Part model, mm, in its own coordinate system. A direction names the side the tool comes from. Round coordinates to 2 decimals unless told otherwise and drop trailing zeros. Loops run counter-clockwise (first coordinate to the right, second up) from the corner with the lowest first, then second, coordinate; pieces in that order, holes last.
(1) Cut at D-D on x = -4. List the corners of the cut face in (y, z).
(2) Mould opens along Z. For faces 1 (the face through (0, 15, -15)), 2 (the face through (-4.01, 12.32, 18.06)), 3 (the face through (0, 25, 0)) say: +Z half, -Z half, draft (parallel to the pull), parting line (faces both ways), or undercut.
(3) Cut at A-A on x = 0. List the corners of the cut face in (y, z) (3 decimals), then the cut area to 3 significant figures.
(4) Tool access for faces 4 (the face through (-0.2, 20.07, 13.78)), 5 (the face through (0, 0, 0)): list every direction of +Z, -Z, +X, -X, +Y, -Y with a clear straight run to the whole face (end or side of a thin tool).
(5) Cut at B-B on y = 6.25. List the corners of the cut face in (x, z), then the cut area to 3 significant figures.
(6) Cut at C-C on x = 12.5. List the corners of the cut face in (y, z).
(7) Probe probe 1 along Z at (x, y) = (0, 17.75) (3 decimals); probe 2 along X at (y, z) = (16.75, 8); probe 3 along Z at (x, y) = (13, 16.25). List the from-to ranges inside material, lowest first.
(8) Flat gauge pins, fed straight in: pin 1 (3 mm diameter, centred on x = 14, y = 15, fed in from +Z); pin 2 (1 mm diameter, centred on x = -13.5, y = 8.5, fed in from -Z); pin 3 (5 mm diameter, centred on x = -5, y = 18.5, fed in from +Z). Where does each tip first touch, or does it go through?
from build123d import *

# Parameters (mm, degrees)
SKETCH1_R           = 18.5
BOSS_EXTRUDE1_DEPTH = 25
SKETCH2_R           = 1.5
CUT_EXTRUDE1_DEPTH  = 10


with BuildPart() as part:
    # Sketch1 → Boss-Extrude1 (new body)
    with BuildSketch(Plane(origin=(0, 0, 0), x_dir=(1, 0, 0), z_dir=(0, 1, 0))):
        Circle(SKETCH1_R)
    extrude(amount=BOSS_EXTRUDE1_DEPTH)

    # Sketch2 → Cut-Extrude1 (cut)
    with BuildSketch(Plane(origin=(0, 25, 0), x_dir=(1, 0, 0), z_dir=(0, 1, 0))):
        with Locations((0, 15.265)):
            Circle(SKETCH2_R)
        with Locations((13.219877789, 7.6325)):
            Circle(SKETCH2_R)
        with Locations((13.219877789, -7.6325)):
            Circle(SKETCH2_R)
        with Locations((0, -15.265)):
            Circle(SKETCH2_R)
        with Locations((-13.219877789, -7.6325)):
            Circle(SKETCH2_R)
        with Locations((-13.219877789, 7.6325)):
            Circle(SKETCH2_R)
    extrude(amount=-CUT_EXTRUDE1_DEPTH, mode=Mode.SUBTRACT)


solid = part.part
Final values:
1. outline: (0, -18.06) - (25, -18.06) - (25, 18.06) - (0, 18.06) - close
2. face 1: undercut
2. face 2: parting line
2. face 3: draft
3. outline: (0, -18.5) - (25, -18.5) - (25, -16.765) - (15, -16.765) - (15, -13.765) - (25, -13.765) - (25, 13.765) - (15, 13.765) - (15, 16.765) - (25, 16.765) - (25, 18.5) - (0, 18.5) - close
3. area: 865 mm2
4. face 4: +Y
4. face 5: +Z, -Z, +X, -X, -Y
5. outline: circle Ø37 at (0, 0)
5. area: 1,080 mm2
6. outline: (0, -13.64) - (25, -13.64) - (25, -8.95) - (15, -8.95) - (15, -6.32) - (25, -6.32) - (25, 6.32) - (15, 6.32) - (15, 8.95) - (25, 8.95) - (25, 13.64) - (0, 13.64) - close
7. probe 1: z = -18.5 to -16.765, -13.765 to 13.765, 16.765 to 18.5
7. probe 2: x = -16.68 to -14.67, -11.77 to 11.77, 14.67 to 16.68
7. probe 3: z = -13.16 to -9.12, -6.15 to 6.15, 9.12 to 13.16
8. pin 1: stops at z = 13.64
8. pin 2: stops at z = -13.16
8. pin 3: stops at z = 18.33
